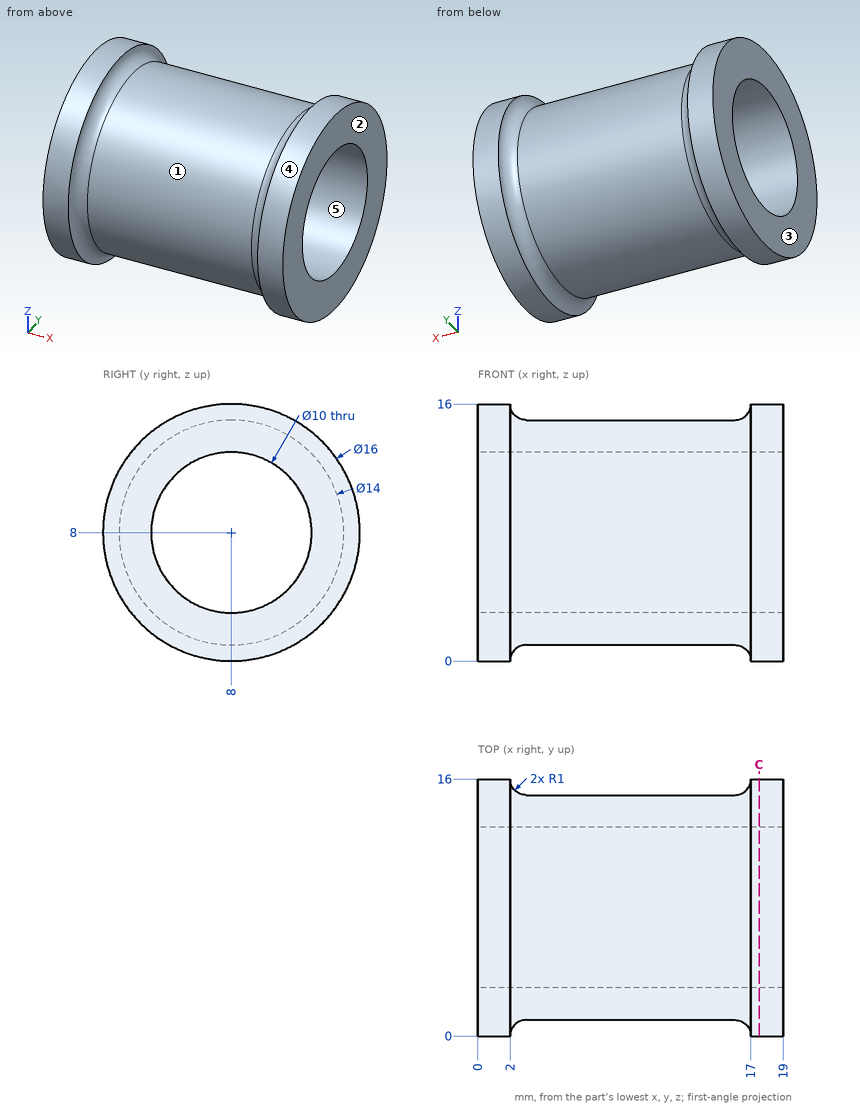
Verification items for this drawing (mm, ordinates from the low corner). A direction names the side the tool comes from. Give positions to 0.01 mm unless a question says otherwise; leave off trailing zeros. Order: outer loops, then holes, each group sorted by start corner. A loop starts at its lowest first (then second) coordinate and runs counter-clockwise, first axis right, second up. Notation, with made-up numbers: M 8.5,-24 L 52.5,-24 A24 cw 52.5,1 Z; hole C 21,75 d2. An arc over 180 degrees is marked long. Use a Markdown table: item, result.
Item 1: Tool access check on the marked faces 1 and 2. Record the directions out of +Z, -Z, +X, -X, +Y, -Y that give a thin tool (end or side, any length) a straight path to the whole face; none if there is none.
Answers follow:
| item | result |
|---|---|
| face 1 | none |
| face 2 | +Z, -Z, +X, +Y, -Y |
Item 2: Draft check along Z on the marked faces 3, 4 and 5. Enter one of: +Z half, -Z half, draft (parallel to the pull), parting line (faces both ways), or undercut.
Answers follow:
| item | result |
|---|---|
| face 3 | draft |
| face 4 | parting line |
| face 5 | undercut |
Item 3: Section check C-C (x = 17.5). Record the cut outline in (y, z).
Answers follow:
| item | result |
|---|---|
| outline | C 8,8 d16; hole C 8,8 d10 |
Item 4: Material ranges on line 1 along Z through (x, y) = (13.5, 8.25); line 2 along Y through (x, z) = (10, 8); line 3 along X through (y, z) = (1.5, 4), recorded low to high.
Answers follow:
| item | result |
|---|---|
| line 1 | z = 1 to 3.01, 12.99 to 15 |
| line 2 | y = 1 to 3, 13 to 15 |
| line 3 | x = 0 to 2.07, 16.93 to 19 |
Item 5: Depth check by flat-ended pin: P1, Ø4, axis at x = 2, z = 2.5, coming from the +Y side; P2, Ø4, axis at x = 9, z = 13.5, coming from the -Y side; P3, Ø2, axis at x = 10.5, y = 3, coming from the +Z side; P4, Ø9, axis at y = 8, z = 8, coming from the -X side. Enter the tip coordinate at first touch or a pass-through.
Answers follow:
| item | result |
|---|---|
| P1 | stops at y = 15.19 |
| P2 | stops at y = 1.94 |
| P3 | stops at z = 13.74 |
| P4 | passes through |
